Could you check a few things on this model? Use its own coordinates, in mm. Face numbers are marked on the shaded views. A direction names the side the tool comes from. Round coordinates to 2 decimals unless told otherwise and drop trailing zeros. Loops run counter-clockwise (first coordinate to the right, second up) from the corner with the lowest first, then second, coordinate; pieces in that order, holes last. Notation, with made-up numbers: (8, 75.5) - (32, 75.5) arc R4 cw to (32, 82.5) - close; hole circle Ø8 at (-6.5, 3.25). An arc over 180 degrees is marked (long way). Answer as CSV lines item,"result". Start each with the question number.
1) We'd pull the mould along X, two halves only. Please class the marked faces 1, 2, 3 and 4: pulls with the +X half, pulls with the -X half, needs draft (parallel to the pull), parting line crosses it, or undercut.
2) Suppose I cut it at D-D, the plane y = 6. Write out the boundary of the cut face in (x, z), then the cut area to 3 significant figures.
3) Which directions (+Z, -Z, +X, -X, +Y, -Y) give clear straight access to the entire face, cutting with the end or side of a thin tool? Please do the marked faces 5 and 6.
4) Please list where these lines run through material, in increasing order: line 1 along X through (y, z) = (1.25, 6.5); line 2 along Z through (x, y) = (2.5, 5.5); line 3 along Y through (x, z) = (1.5, 7.25).
5) I'm going to push flat-ended pins straight in: pin 1 Ø1.8 at (x, z) = (5, 4.5) entering from +Y; pin 2 Ø3 at (x, z) = (1, 4) entering from +Y. Where does each tip first touch, or does it pass through?
6) Suppose I cut it at A-A, the plane z = 2.5. Write out the boundary of the cut face in (x, y), then the cut area to 3 significant figures.
7) Suppose I cut it at B-B, the plane y = 8. Write out the boundary of the cut face in (x, z).
8) Suppose I cut it at C-C, the plane x = 4.75. Write out the boundary of the cut face in (y, z).
```python
from build123d import *

# Parameters (mm, degrees)
F1_DEPTH = 8
F3_START = 1.7
F2_W     = 6
F2_H     = 9
F3_DEPTH = 20.7
F4_R     = 1
F5_DEPTH = 19.8


with BuildPart() as f1:
    # F0 (on Right) → F1 (new body)
    with BuildSketch(Plane.YZ):
        Polygon((0, 10), (0, 0), (10, 0), align=None)
    extrude(amount=F1_DEPTH)

    # F2 (on Top) → F3 (cut)
    with BuildSketch(Plane.XY.offset(F3_START)):
        with Locations((4.0581296198, 5.5038969816)):
            Rectangle(F2_W, F2_H)
    extrude(amount=F3_DEPTH, mode=Mode.SUBTRACT)

    # F4 (on Top) → F5 (cut)
    with BuildSketch(Plane.XY):
        with Locations((4.1189291514, 5.1976959221)):
            Circle(F4_R)
    extrude(amount=F5_DEPTH, mode=Mode.SUBTRACT)


solid = f1.part
```
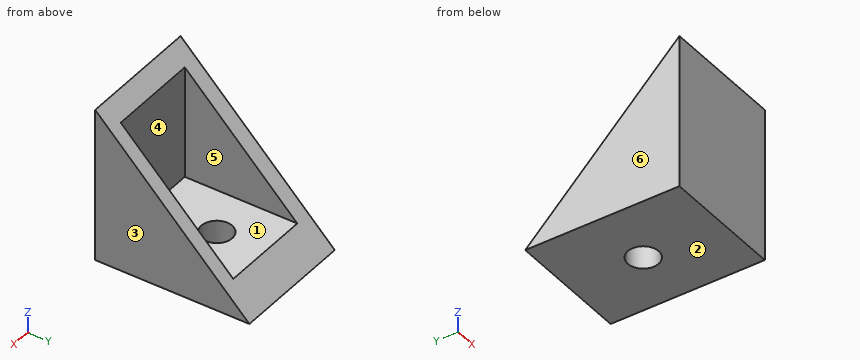
Filled sheet:
1,face 1,"undercut"
1,face 2,"needs draft"
1,face 3,"pulls with the +X half"
1,face 4,"undercut"
2,outline,"(0, 0) - (3.52, 0) - (3.52, 1.7) - (1.06, 1.7) - (1.06, 4) - (0, 4) - close; (4.72, 0) - (8, 0) - (8, 4) - (7.06, 4) - (7.06, 1.7) - (4.72, 1.7) - close"
2,area,"16.2 mm²"
3,face 5,"+Z, +Y"
3,face 6,"+Z, -Z, -X, +Y, -Y"
4,line 1,"0 to 1.06, 7.06 to 8"
4,line 2,"0 to 1.7"
4,line 3,"0 to 1"
5,pin 1,"y = 1"
5,pin 2,"y = 7.5"
6,outline,"(0, 0) - (8, 0) - (8, 7.5) - (7.06, 7.5) - (7.06, 1) - (1.06, 1) - (1.06, 7.5) - (0, 7.5) - close"
6,area,"21.0 mm²"
7,outline,"(0, 0) - (8, 0) - (8, 2) - (7.06, 2) - (7.06, 1.7) - (1.06, 1.7) - (1.06, 2) - (0, 2) - close"
8,outline,"(0, 0) - (4.42, 0) - (4.42, 1.7) - (1, 1.7) - (1, 9) - (0, 10) - close; (5.97, 0) - (10, 0) - (8.3, 1.7) - (5.97, 1.7) - close"
